Here's how the part is built. I have some questions about the finished solid (model axes, mm). A direction names the side the tool comes from. Coordinates: 2 decimals unless noted, no trailing zeros. Write each loop counter-clockwise with the first axis right and the second up, starting at its lowest first coordinate (ties: lowest second). Pieces come first, ordered by that corner, then holes. Notation, with made-up numbers: (60, -16) -> (93, -16) arc R10 cw to (93, -6) -> close; hole circle Ø4 at (60.5, 19). An arc over 180 degrees is marked (long way). Use a Markdown table: item, result. Add a question column.
```python
from build123d import *

# Parameters (mm, degrees)
SKETCH1_R             = 4
SKETCH1_R_2           = 2
BOSS_EXTRUDE2_DEPTH   = 6.038447986
BOSS_EXTRUDE2_2_DEPTH = 6.038447986
BOSS_EXTRUDE2_3_DEPTH = 6.038447986
BOSS_EXTRUDE2_4_DEPTH = 6.038447986
BOSS_EXTRUDE4_DEPTH   = 3
SKETCH2_W             = 8
SKETCH2_H             = 10
SKETCH2_R             = 2
BOSS_EXTRUDE3_DEPTH   = 5
SKETCH1_4_R           = 2
SKETCH1_4_R_2         = 13
CUT_EXTRUDE1_DEPTH    = 10


with BuildPart() as part:
    # Sketch1 → Boss-Extrude2 (new body)
    with BuildSketch(Plane.XY):
        with Locations((49, 35.83595021)):
            Circle(SKETCH1_R)
        with Locations((49, 35.83595021)):
            Circle(SKETCH1_R_2, mode=Mode.SUBTRACT)
    extrude(amount=BOSS_EXTRUDE2_DEPTH)



with BuildPart() as body_2:
    # Sketch1 → Boss-Extrude2 2 (new body)
    with BuildSketch(Plane.XY):
        with Locations((49, 7.83595021)):
            Circle(SKETCH1_R)
        with Locations((49, 7.83595021)):
            Circle(SKETCH1_R_2, mode=Mode.SUBTRACT)
    extrude(amount=BOSS_EXTRUDE2_2_DEPTH)


with BuildPart() as body_3:
    # Sketch1 → Boss-Extrude2 3 (new body)
    with BuildSketch(Plane.XY):
        with Locations((9, 7.83595021)):
            Circle(SKETCH1_R)
        with Locations((9, 7.83595021)):
            Circle(SKETCH1_R_2, mode=Mode.SUBTRACT)
    extrude(amount=BOSS_EXTRUDE2_3_DEPTH)


with BuildPart() as body_4:
    # Sketch1 → Boss-Extrude2 4 (new body)
    with BuildSketch(Plane.XY):
        with Locations((9, 35.83595021)):
            Circle(SKETCH1_R)
        with Locations((9, 35.83595021)):
            Circle(SKETCH1_R_2, mode=Mode.SUBTRACT)
    extrude(amount=BOSS_EXTRUDE2_4_DEPTH)


with BuildPart() as part_1:
    add(part.part)

    add(body_2.part)  # Boss-Extrude4 merges body 2

    add(body_3.part)  # Boss-Extrude4 merges body 3

    add(body_4.part)  # Boss-Extrude4 merges body 4
    # Sketch3 → Boss-Extrude4 (add)
    with BuildSketch(Plane.XY.offset(6.038447986)):
        Polygon((-8, 6.83595021), (-8, -9.86404979), (66, -9.86404979), (66, 6.83595021), (58, 6.83595021), (58, 41.83595021), (0, 41.83595021), (0, 6.83595021), align=None)
    extrude(amount=BOSS_EXTRUDE4_DEPTH)

    # Sketch2 → Boss-Extrude3 (add)
    # profile 1 of 2: a face of its own
    with BuildSketch(Plane(origin=(0, 1.83595021, 0), x_dir=(1, 0, 0), z_dir=(0, 1, 0))):
        with Locations((-4, -1.038447986)):
            Rectangle(SKETCH2_W, SKETCH2_H)
        with Locations(Location((-4, -1.038447986, 0), (0, 0, 270))):
            Circle(SKETCH2_R, mode=Mode.SUBTRACT)
    # profile 2 of 2: a face of its own
    with BuildSketch(Plane(origin=(0, 1.83595021, 0), x_dir=(1, 0, 0), z_dir=(0, 1, 0))):
        with Locations((62, -1.038447986)):
            Rectangle(SKETCH2_W, SKETCH2_H)
        with Locations(Location((62, -1.038447986, 0), (0, 0, 270))):
            Circle(SKETCH2_R, mode=Mode.SUBTRACT)
    extrude(amount=BOSS_EXTRUDE3_DEPTH)

    # Sketch1<4> → Cut-Extrude1 (cut)
    with BuildSketch(Plane.XY):
        with Locations((9, 35.83595021)):
            Circle(SKETCH1_4_R)
        with Locations((9, 7.83595021)):
            Circle(SKETCH1_4_R)
        with Locations((49, 35.83595021)):
            Circle(SKETCH1_4_R)
        with Locations((38.5, 21.83595021)):
            Circle(SKETCH1_4_R_2)
        with Locations((49, 7.83595021)):
            Circle(SKETCH1_4_R)
    extrude(amount=CUT_EXTRUDE1_DEPTH, mode=Mode.SUBTRACT)


solid = part_1.part
```
Q1. Suppose I cut it at B-B, the plane z = 4.5. State how many separate pieces and enclosed holes the cut face has, and give its area (3 significant figures).
Q2. Will these pins go through, and if not, where does the flat tip stop? pin 1 (2 mm diameter, centred on x = 12, z = 0.5, fed in from -Y); pin 2 (4 mm diameter, centred on x = -5.5, z = 4.5, fed in from +Y); pin 3 (2.5 mm diameter, centred on x = 62, z = 1.04, fed in from -Y); pin 4 (9 mm diameter, centred on x = 10, y = 37, fed in from -Z).
Q3. Suppose I cut it at A-A, the plane x = 38.5. Write out the boundary of the cut face in (y, z).
Q4. Suppose I cut it at D-D, the plane y = 27.5. Write out the boundary of the cut face in (x, z).
Q5. Please list where these lines run through material, in increasing order: line 1 (Y direction, x = 9, z = 2.75); line 2 (Y direction, x = 49, z = 6.25); line 3 (X direction, y = 37, z = 5).
Q6. Thinking about a two-plate mould opening in Y: for faces 5 (the flat face through (7, 7, 0)), 6 (the flat face through (-6, 1.836, 0)), 7 (the cylindrical face through (45.004, 8.012, 2.977)), 8 (the flat face through (-4, 6.836, 4)), which applies, released by +Y, released by -Y, zero draft, split by the parting line, or undercut?
Q7. Suppose I cut it at C-C, the plane x = 9. Write out the boundary of the cut face in (y, z), and give its area (3 significant figures).
Q8. Which directions (+Z, -Z, +X, -X, +Y, -Y) give clear straight access to the entire face, cutting with the end or side of a thin tool? Please do faces 1 (the flat face through (62, 6.836, 4)), 2 (the flat face through (58, 4, 1)), 3 (the flat face through (60, 1.836, 0)), 4 (the flat face through (0, 25, 8)).
Answer key:
| question | item | result |
|---|---|---|
| 1 | separate pieces | 6 |
| 1 | enclosed holes | 4 |
| 1 | area | 231 mm^2 |
| 2 | pin 1 | stops at y = 4.37 |
| 2 | pin 2 | stops at y = 6.84 |
| 2 | pin 3 | passes through |
| 2 | pin 4 | stops at z = 0 |
| 3 | outline | (-9.86, 6.04) -> (8.84, 6.04) -> (8.84, 9.04) -> (-9.86, 9.04) -> close; (34.84, 6.04) -> (41.84, 6.04) -> (41.84, 9.04) -> (34.84, 9.04) -> close |
| 4 | outline | (0, 6.04) -> (26.8, 6.04) -> (26.8, 9.04) -> (0, 9.04) -> close; (50.2, 6.04) -> (58, 6.04) -> (58, 9.04) -> (50.2, 9.04) -> close |
| 5 | line 1 | y = 3.84 to 5.84, 9.84 to 11.84, 31.84 to 33.84, 37.84 to 39.84 |
| 5 | line 2 | y = -9.86 to 5.84, 9.84 to 14.17, 29.5 to 33.84, 37.84 to 41.84 |
| 5 | line 3 | x = 5.17 to 7.37, 10.63 to 12.83, 45.17 to 47.37, 50.63 to 52.83 |
| 6 | face 5 | zero draft |
| 6 | face 6 | released by -Y |
| 6 | face 7 | undercut |
| 6 | face 8 | released by +Y |
| 7 | outline | (-9.86, 6.04) -> (3.84, 6.04) -> (3.84, 0) -> (5.84, 0) -> (5.84, 9.04) -> (-9.86, 9.04) -> close; (9.84, 0) -> (11.84, 0) -> (11.84, 6.04) -> (31.84, 6.04) -> (31.84, 0) -> (33.84, 0) -> (33.84, 9.04) -> (9.84, 9.04) -> close; (37.84, 0) -> (39.84, 0) -> (39.84, 6.04) -> (41.84, 6.04) -> (41.84, 9.04) -> (37.84, 9.04) -> close |
| 7 | area | 179 mm^2 |
| 8 | face 1 | +Z, -Z, +X, +Y |
| 8 | face 2 | -Z, +Y, -Y |
| 8 | face 3 | -Z, +X, -X, -Y |
| 8 | face 4 | +Z, -Z, -X, +Y |
